```python
from build123d import *

# Parameters (mm, degrees)
SKETCH3_R           = 41.5
BOSS_EXTRUDE1_DEPTH = 2.5
FILLET1_R           = 5


# Read off the part's stored shape, not the designer's step: Loft-Thin1
with BuildPart() as part:
    # Loft-Thin1 outline → Loft-Thin1 (revolve)
    with BuildSketch(Plane.XY):
        Polygon((43.5, 96.5), (41.499758397, 96.5), (42.999758397, 0), (45, 0), align=None)
    revolve(axis=Axis((0, 0, 0), (0, 1, 0)))

    # Sketch3 → Boss-Extrude1 (add)
    with BuildSketch(Plane(origin=(0, 96.5, 0), x_dir=(1, 0, 0), z_dir=(0, 1, 0))):
        with Locations(Location((0, 0, 0), (0, 0, 270))):
            Circle(SKETCH3_R)
    extrude(amount=-BOSS_EXTRUDE1_DEPTH)

    # Fillet1
    fillet1_edges = [part.edges().sort_by_distance(p)[0] for p in [
        (-43.5, 96.5, 0),
    ]]
    fillet(fillet1_edges, radius=FILLET1_R)


solid = part.part
```
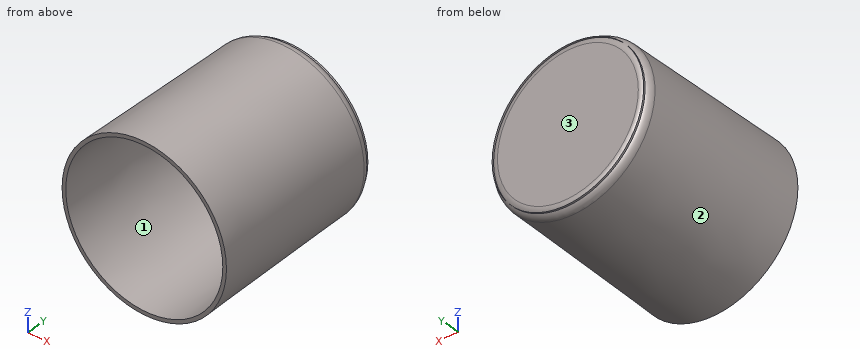
Source: CAD feature listing. Evaluate the final solid. Frame: model axes, mm. Face numbers are marked on the shaded views. Coordinates: 2 decimals unless noted, no trailing zeros. Loops run counter-clockwise (first coordinate to the right, second up) from the corner with the lowest first, then second, coordinate; pieces in that order, holes last. Notation, with made-up numbers: (56, 48) - (68, 48) arc R12 ccw to (68, 61) - close; hole circle Ø9 at (-26.5, -39.75). An arc over 180 degrees is marked (long way). Answer as CSV lines item,"result".
1. Section D-D (y = 39). Return loops of the section in (x, z), then the cut area to 3 significant figures.
Established:
outline,"circle Ø88.79 at (0, 0); hole circle Ø84.79 at (0, 0)"
area,"545 mm2"
2. Section C-C (y = 71.5). Return loops of the section in (x, z), then the cut area to 3 significant figures.
Established:
outline,"circle Ø87.78 at (0, 0); hole circle Ø83.78 at (0, 0)"
area,"539 mm2"
3. Ray query, line 1 (Y direction, x = -6, z = -35.5); line 2 (Z direction, x = 31.5, y = 49.5); line 3 (X direction, y = 70, z = -28). Return the intervals inside material, ascending.
Established:
line 1,"y = 94 to 96.5"
line 2,"z = -31.05 to -28.13, 28.13 to 31.05"
line 3,"x = -33.83 to -31.19, 31.19 to 33.83"
4. Contact query for flat-ended pins moving along their axis: pin 1 (1.5 mm diameter, centred on x = 14, y = 86.5, fed in from -Z); pin 2 (5 mm diameter, centred on x = 15, y = 84.5, fed in from +Z); pin 3 (2 mm diameter, centred on x = -31.5, y = 45, fed in from -Z). Output: stop coordinate, or through.
Established:
pin 1,"stops at z = -41.6"
pin 2,"stops at z = 41.86"
pin 3,"stops at z = -32.13"
5. Mould query, pull axis X, two halves, no side actions, for the marked faces 1, 2 and 3. Classes: released by +X, released by -X, zero draft, split by the parting line, or undercut.
Established:
face 1,"undercut"
face 2,"split by the parting line"
face 3,"zero draft"
